Verification items for the finished model (mm, model axes). A direction names the side the tool comes from. Coordinates: 2 decimals unless noted, no trailing zeros. Loops run counter-clockwise (first coordinate to the right, second up) from the corner with the lowest first, then second, coordinate; pieces in that order, holes last. Notation, with made-up numbers: (47.5, 67) -> (80.5, 67) arc R25 cw to (80.5, 100) -> close; hole circle Ø2 at (74, 67.25). An arc over 180 degrees is marked (long way). Answer as a JSON object with one key per item and string values. Group by question number.
Q1. Cross-section at C-C on y = 17. Record the boundary of the cut face in (x, z), and give its area (3 significant figures).
Q2. Set-up check for faces 5 (the flat face through (6.034, 2.712, 3.549)), 6 (the cylindrical face through (-11.99, 13.46, 0.53)): record each of +Z, -Z, +X, -X, +Y, -Y from which the full face is reachable in a straight line by a thin tool's end or side.
Q3. Release check for a two-part mould opening along X. For faces 1 (the flat face through (-6.034, 2.712, -3.549)), 2 (the flat face through (0, 0, -8)), 3 (the conical face through (-1.98, 7.81, 15.06)), 4 (the cylindrical face through (-3.14, 2.46, -9.24)) record: released by +X, released by -X, zero draft, split by the parting line, or undercut.
Q4. Gauge pin test, flat ends, axial feed: pin 1 Ø2.5 at (x, z) = (-3.43, 10.56) entering from +Y; pin 2 Ø6 at (x, y) = (-6.5, 15.5) entering from +Z; pin 3 Ø6 at (y, z) = (16.5, -8.5) entering from -X. Record the tip position at first contact, or that the pin passes through.
Q5. Scan lines: L1, parallel to Z at x = 0, y = 13; L2, parallel to X at y = 3.75, z = -1. Record each from-to range of solid material in increasing order.
Q6. Cross-section at B-B on y = 14. Record the boundary of the cut face in (x, z).
Autodesk Inventor part; units mm, degrees
ref_plane "YZ Plane" through (0, 0, 0) normal (1, 0, 0) x (0, 1, 0)
ref_plane "XZ Plane" through (0, 0, 0) normal (0, 1, 0) x (-1, 0, 0)
ref_plane "XY Plane" through (0, 0, 0) normal (0, 0, 1) x (1, 0, 0)
sketch "Sketch1" plane through (0, 0, 0) normal (0, 1, 0) x (-1, 0, 0)
  circle A0 centre (0, 0) radius 18
  line L0 (10.3065, -1.0922) -> (4.2236, -9.4646)
  line L1 (2.1462, -10.1396) -> (-7.6962, -6.9416)
  line L2 (-8.9801, -5.1744) -> (-8.9801, 5.1744)
  line L3 (-7.6962, 6.9416) -> (2.1462, 10.1396)
  line L4 (4.2236, 9.4646) -> (10.3065, 1.0922)
  circle A1 centre (3.4301, 10.5567) radius 1.35
  circle A2 centre (11.1, 0) radius 1.35
  circle A3 centre (-8.9801, 6.5244) radius 1.35
  circle A4 centre (-8.9801, -6.5244) radius 1.35
  circle A5 centre (3.4301, -10.5567) radius 1.35
  arc A6 (11.0179, 1.3475) -> (4.6863, 10.0622) centre (0, 0) ccw
  arc A7 (4.6863, -10.0622) -> (11.0179, -1.3475) centre (0, 0) ccw
  arc A8 (-8.1216, -7.5663) -> (2.1232, -10.8951) centre (0, 0) ccw
  arc A9 (2.1232, 10.8951) -> (-8.1216, 7.5663) centre (0, 0) ccw
  arc A10 (-9.7057, 5.386) -> (-9.7057, -5.386) centre (0, 0) ccw
  dimension "d0" = 36
  dimension "d2" = 2.7
  dimension "d3" = 2.7
  dimension "d4" = 2.7
  dimension "d5" = 2.7
  dimension "d6" = 2.7
extrude "Extrusion1" add sketch "Sketch1" along normal blind 5 contours A0 | A2 A7 A5 L0 | L0 A5 L1 A4 L2 A3 L3 A1 L4 A2 | L4 A1 A6 A2 | A5 A8 A4 L1 | L3 A3 A9 A1 | A10 A3 L2 A4
sketch "Sketch2" plane through (0, 5, 0) normal (0, 1, 0) x (1, 0, 0)
  circle A0 centre (0, 0) radius 18
  circle A1 centre (0, 0) radius 15
  point P0 (2.5, -14.7902)
  point P1 (2.5, 14.7902)
  dimension "d9" = 30
extrude "Extrusion2" add sketch "Sketch2" along normal blind 6 contours A1
sketch "Sketch3" plane through (0, 0, 0) normal (0, -1, 0) x (1, 0, 0)
  circle A0 centre (0, 0) radius 18
  line L0 (-8.0829, 0) -> (-4.0415, 7)
  line L1 (-4.0415, 7) -> (4.0415, 7)
  line L2 (4.0415, 7) -> (8.0829, 0)
  line L3 (8.0829, 0) -> (4.0415, -7)
  line L4 (4.0415, -7) -> (-4.0415, -7)
  line L5 (-4.0415, -7) -> (-8.0829, 0)
  dimension "d23" = 14
extrude "Extrusion3" cut sketch "Sketch3" against normal blind 5.5 contours L0 L1 L2 L3 L4 L5
sketch "Sketch4" plane through (0, 5.5, 0) normal (0, -1, 0) x (1, 0, 0)
  circle A0 centre (0, 0) radius 4.5
  dimension "d26" = 9
extrude "Extrusion4" cut sketch "Sketch4" against normal blind 9
chamfer "Chamfer1" distance 3 angle 45 2 edges at (-15, 5, 0) (-15, 11, 0)
sketch "Sketch5" plane through (0, 11, 0) normal (0, 1, 0) x (1, 0, 0)
  circle A0 centre (0, 0) radius 4.5
  circle A1 centre (0, 0) radius 12
extrude "Extrusion5" add sketch "Sketch5" along normal blind 8
chamfer "Chamfer2" distance 3 angle 45 1 edges at (-12, 19, 0)
equation "\"BendRadius\" = Thickness"
equation "\"BendReliefWidth\" = Thickness"
equation "\"BendReliefDepth\" = 0.5 * Thickness"
equation "\"CornerReliefSize\" = 4 * Thickness"
equation "\"MinimumRemnant\" = 2 * Thickness"
equation "\"TransitionRadius\" = BendRadius"
equation "\"JacobiRadiusSize\" = BendRadius"
equation "\"GapSize\" = Thickness"
properties part number "motorSupportNew1 modified2"
Computed values:
{
 "1": {"outline": "circle Ø22 at (0, 0); hole circle Ø9 at (0, 0)", "area": "317 mm²"},
 "2": {"face 5": "-Y", "face 6": "+Y"},
 "3": {"face 1": "undercut", "face 2": "zero draft", "face 3": "split by the parting line", "face 4": "undercut"},
 "4": {"pin 1": "stops at y = 18.15", "pin 2": "stops at z = 11.48", "pin 3": "stops at x = -10.64"},
 "5": {"L1": "z = -12 to -4.5, 4.5 to 12", "L2": "x = -17.97 to -12.01, -10.19 to -7.51, 7.51 to 17.97"},
 "6": {"outline": "circle Ø24 at (0, 0); hole circle Ø9 at (0, 0)"}
}
